```python
from build123d import *

# Parameters (mm, degrees)
SKETCH_W        = 55
SKETCH_H        = 60
PAD_DEPTH       = 14
SKETCH001_R     = 7.6
POCKET_DEPTH    = 60.001
SKETCH002_R     = 1.75
POCKET001_DEPTH = 14.001
POCKET002_DEPTH = 12
SKETCH004_R     = 2.25
POCKET003_DEPTH = 14.001
SKETCH008_R     = 4.1
POCKET005_DEPTH = 20
SKETCH010_W     = 20
SKETCH010_H     = 25
POCKET006_DEPTH = 5
CHAMFER_SIZE    = 3
SKETCH011_R     = 2.9
POCKET007_DEPTH = 3.5


with BuildPart() as part:
    # Sketch → Pad (new body)
    with BuildSketch(Plane.XY):
        with Locations((17.5, 0)):
            Rectangle(SKETCH_W, SKETCH_H)
    extrude(amount=PAD_DEPTH)

    # Sketch001 → Pocket (cut, through all)
    with BuildSketch(Plane.XZ.offset(30)):
        with Locations((0, 14)):
            Circle(SKETCH001_R)
    extrude(amount=-POCKET_DEPTH, mode=Mode.SUBTRACT)

    # Sketch002 → Pocket001 (cut, through all)
    with BuildSketch(Plane.XY.offset(14)):
        with Locations((-6, 27)):
            Circle(SKETCH002_R)
        with Locations((36, 27)):
            Circle(SKETCH002_R)
        with Locations((-6, -27)):
            Circle(SKETCH002_R)
        with Locations((36, -27)):
            Circle(SKETCH002_R)
        with Locations((6, 27)):
            Circle(SKETCH002_R)
        with Locations((6, -27)):
            Circle(SKETCH002_R)
        with Locations((6, 0)):
            Circle(SKETCH002_R)
        with Locations((-6, 0)):
            Circle(SKETCH002_R)
        with Locations((36, -13)):
            Circle(SKETCH002_R)
        with Locations((36, 13)):
            Circle(SKETCH002_R)
    extrude(amount=-POCKET001_DEPTH, mode=Mode.SUBTRACT)

    # Sketch003 → Pocket002 (cut)
    with BuildSketch(Plane.XY.offset(14)):
        with BuildLine():
            Line((10, 35), (10, -35))
            Line((10, -35), (28, -35))
            Line((28, -35), (28, -14.916198))
            ThreePointArc((28, -14.916198), (30.841983, -12.965458), (32.599342, -10))
            Line((32.599342, -10), (52.599342, -10))
            Line((52.599342, -10), (52.599342, 10))
            Line((52.599342, 10), (32.599342, 10))
            ThreePointArc((32.599342, 10), (30.841983, 12.965458), (28, 14.916198))
            Line((28, 14.916198), (28, 35))
            Line((28, 35), (10, 35))
        make_face()
    extrude(amount=-POCKET002_DEPTH, mode=Mode.SUBTRACT)

    # Sketch004 → Pocket003 (cut, through all)
    with BuildSketch(Plane(origin=(0, 0, 0), x_dir=(1, 0, 0), z_dir=(0, 0, -1))):
        with Locations((25, 7.5)):
            Circle(SKETCH004_R)
        with Locations((25, -7.5)):
            Circle(SKETCH004_R)
    extrude(amount=-POCKET003_DEPTH, mode=Mode.SUBTRACT)

    # Sketch008 → Pocket005 (cut)
    with BuildSketch(Plane.YZ.offset(45)):
        with Locations((-20, 14)):
            Circle(SKETCH008_R)
        with Locations((20, 14)):
            Circle(SKETCH008_R)
    extrude(amount=-POCKET005_DEPTH, mode=Mode.SUBTRACT)

    # Sketch010 → Pocket006 (cut)
    with BuildSketch(Plane.YZ.offset(45)):
        with Locations((0, 5.473744)):
            Rectangle(SKETCH010_W, SKETCH010_H)
    extrude(amount=-POCKET006_DEPTH, mode=Mode.SUBTRACT)

    # Chamfer
    chamfer_edges = [part.edges().sort_by_distance(p)[0] for p in [
        (45, -10, 8),
        (45, 10, 8),
    ]]
    chamfer(chamfer_edges, length=CHAMFER_SIZE)

    # Sketch011 → Pocket007 (cut)
    with BuildSketch(Plane(origin=(0, 0, 0), x_dir=(1, 0, 0), z_dir=(0, 0, -1))):
        with Locations((36, 27)):
            Circle(SKETCH011_R)
        with Locations((36, 13)):
            Circle(SKETCH011_R)
        with Locations((36, -13)):
            Circle(SKETCH011_R)
        with Locations((36, -27)):
            Circle(SKETCH011_R)
        with Locations((-6, 27)):
            Circle(SKETCH011_R)
        with Locations((6, 27)):
            Circle(SKETCH011_R)
        with Locations((-6, 0)):
            Circle(SKETCH011_R)
        with Locations((6, 0)):
            Circle(SKETCH011_R)
        with Locations((-6, -27)):
            Circle(SKETCH011_R)
        with Locations((6, -27)):
            Circle(SKETCH011_R)
    extrude(amount=-POCKET007_DEPTH, mode=Mode.SUBTRACT)


solid = part.part
```
Check sheet for the modelled part. Datum: model origin and axes. Units: mm. A direction names the side the tool comes from. Coordinates: 2 decimals unless noted, no trailing zeros. Order: outer loops, then holes, each group sorted by start corner. A loop starts at its lowest first (then second) coordinate and runs counter-clockwise, first axis right, second up. Notation, with made-up numbers: M -13.75,12 L -7.75,12 A14 ccw -7.75,27 Z; hole C 40,69 d6. An arc over 180 degrees is marked long. One line per question, with ' | ' between items. Start each with the question number.
Item 1: Material ranges on line 1 (X direction, y = 0, z = 1); line 2 (X direction, y = -27, z = 2.1); line 3 (Y direction, x = 36, z = 9.5), recorded low to high.
Item 2: Mould release check, pull along X, two halves, no side actions. Record for faces 5 (the flat face through (-10, 0, 7)), 6 (the flat face through (36, 15, 3.5)), 7 (the cylindrical face through (36.6, 19.9, 9.9)): pulls with the +X half, pulls with the -X half, needs draft (parallel to the pull), parting line crosses it, or undercut.
Item 3: Sectioned sample at C-C on x = 41. Record the cut outline in (y, z), and give its area (3 significant figures).
Item 4: Gauge pin test, flat ends, axial feed: P1, Ø2, axis at x = 36, y = -27, coming from the -Z side; P2, Ø1.5, axis at x = 32.5, y = -7, coming from the +Z side; P3, Ø5.5, axis at x = -6, y = -27, coming from the -Z side. Record the tip position at first contact, or that the pin passes through.
Item 5: Access from +Z, -Z, +X, -X, +Y, -Y to the whole of each face (thin tool, end or side, straight path). Record for faces 1 (the cylindrical face through (36.6, -20.1, 9.9)), 2 (the flat face through (10, 0, 8)), 3 (the flat face through (21, 0, 2)), 4 (the flat face through (-6, 29, 3.5)).
Item 6: Sectioned sample at A-A on y = -7.5. Record the cut outline in (x, z), and give its area (3 significant figures).
Item 7: Sectioned sample at B-B on x = 25. Record the cut outline in (y, z).
Item 8: Sectioned sample at D-D on y = -27. Count the separate pieces of the cut face and the enclosed holes in it, and give its area (3 significant figures).
Answer below:
1) line 1: x = -10 to -8.9, -3.1 to 3.1, 8.9 to 40 | line 2: x = -10 to -8.9, -3.1 to 3.1, 8.9 to 10, 28 to 33.1, 38.9 to 45 | line 3: y = -30 to -28.75, -25.25 to -14.75, -11.25 to -10, 10 to 11.25, 14.75 to 25.25, 28.75 to 30
2) face 5: pulls with the -X half | face 6: undercut | face 7: needs draft
3) outline: M -30,0 L -10,0 L -10,14 L -15.9,14 A4.1 cw -24.1,14 L -30,14 Z; M 10,0 L 30,0 L 30,14 L 24.1,14 A4.1 cw 15.9,14 L 10,14 Z | area: 507 mm^2
4) P1: passes through | P2: stops at z = 2 | P3: stops at z = 3.5
5) face 1: +Z, +X | face 2: +Z, +Y, -Y | face 3: +Z | face 4: -Z
6) outline: M -10,0 L 22.75,0 L 22.75,2 L 10,2 L 10,14 L 7.6,14 A7.6 cw -7.6,14 L -10,14 Z; M 27.25,0 L 40,0 L 40,2 L 27.25,2 Z | area: 240 mm^2
7) outline: M -30,0 L -9.75,0 L -9.75,2 L -30,2 Z; M -5.25,0 L 5.25,0 L 5.25,2 L -5.25,2 Z; M 9.75,0 L 30,0 L 30,2 L 9.75,2 Z
8) separate pieces: 4 | enclosed holes: 0 | area: 322 mm^2
